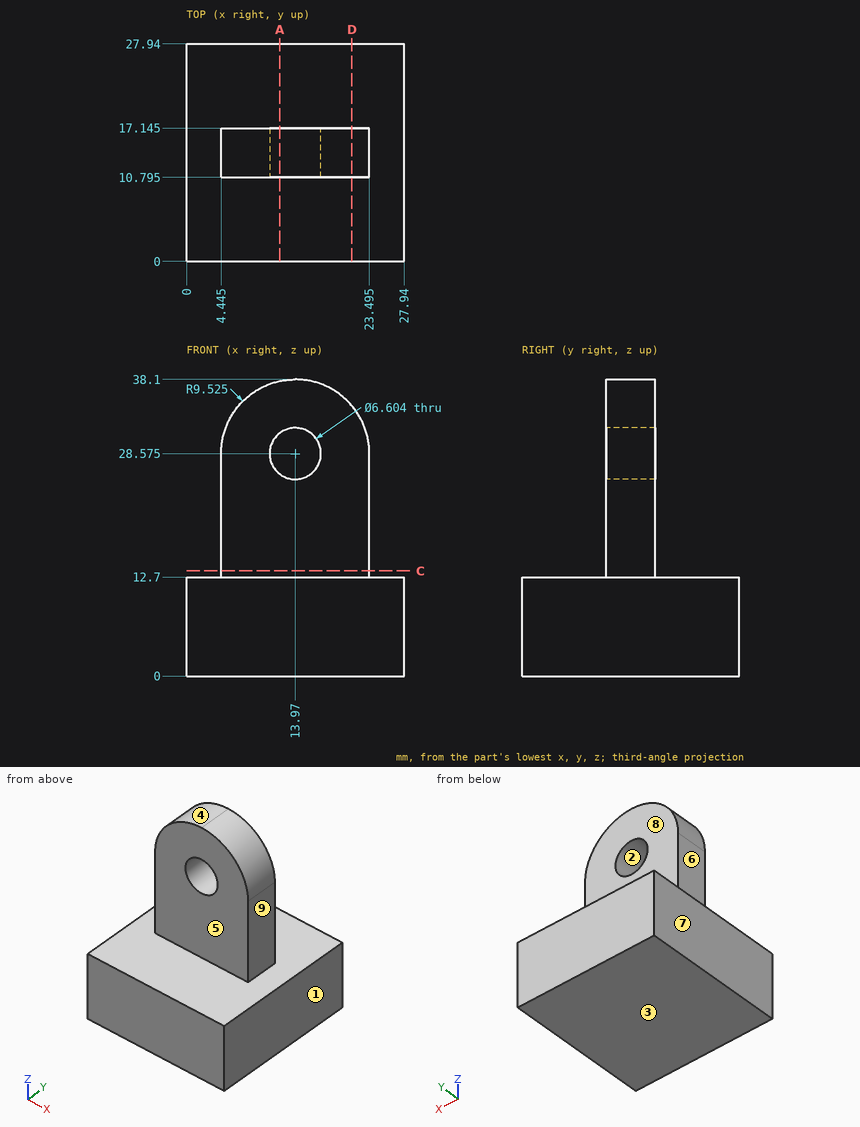
Study the drawing (mm; zero at the part's minimum x, y, z) and answer. A direction names the side the tool comes from. Give positions to 0.01 mm unless a question says otherwise; leave off trailing zeros. Loops run counter-clockwise (first coordinate to the right, second up) from the corner with the lowest first, then second, coordinate; pieces in that order, holes last. Notation, with made-up numbers: (82.25, 88) - (112.25, 88) arc R23 cw to (112.25, 113) - close; hole circle Ø2 at (-3, 52). An arc over 180 degrees is marked (long way). Return JSON: item names as keys, results as strings. Group by question number.
1. Straight lines are drawn through the part: line 1 (Z direction, x = 13.97, y = 14.75); line 2 (Y direction, x = 10.25, z = 31) (3 decimals); line 3 (Z direction, x = 9.75, y = 5.5). For each, find the intervals that lie inside material, in ascending order. Write a range as [from, to].
2. Which of the six approach directions +Z, -Z, +X, -X, +Y, -Y give full straight-line access (tool end or side, diameter ignored) to the marked faces 5, 6, 7, 8 and 9?
3. Given pin 1 Ø4 at (x, y) = (12.5, 7.5) entering from -Z; pin 2 Ø1.9 at (y, z) = (14, 21) entering from -X (3 decimals); pin 3 Ø4 at (x, y) = (19.5, 8) entering from +Z; pin 4 Ø5.5 at (x, z) = (15.5, 31) entering from -Y (3 decimals), each flat-ended and moving along its own axis, determine where each tip first touches the part or whether it passes through.
4. Find section D-D (x = 21.25). Write down the section's boundary in (y, z) (3 decimals).
5. Determine the mould class of the marked faces 1, 2, 3 and 4 for opening direction X: pulls with the +X half, pulls with the -X half, needs draft (parallel to the pull), parting line crosses it, or undercut.
6. Find section A-A (x = 12). Write down the section's boundary in (y, z) (3 decimals).
7. Find section C-C (z = 13.5). Write down the section's boundary in (x, y) (3 decimals).
Verdict:
{
 "1": {"line 1": "z = [0, 25.27], [31.88, 38.1]", "line 2": "y = [10.795, 17.145]", "line 3": "z = [0, 12.7]"},
 "2": {"face 5": "+Z, +X, -X, -Y", "face 6": "+Z, -X, +Y, -Y", "face 7": "+Z, -Z, -X, +Y, -Y", "face 8": "+Z, +X, -X, +Y", "face 9": "+Z, +X, +Y, -Y"},
 "3": {"pin 1": "stops at z = 0", "pin 2": "stops at x = 4.445", "pin 3": "stops at z = 12.7", "pin 4": "stops at y = 10.795"},
 "4": {"outline": "(0, 0) - (27.94, 0) - (27.94, 12.7) - (17.145, 12.7) - (17.145, 34.717) - (10.795, 34.717) - (10.795, 12.7) - (0, 12.7) - close"},
 "5": {"face 1": "pulls with the +X half", "face 2": "undercut", "face 3": "needs draft", "face 4": "pulls with the -X half"},
 "6": {"outline": "(0, 0) - (27.94, 0) - (27.94, 12.7) - (17.145, 12.7) - (17.145, 25.925) - (10.795, 25.925) - (10.795, 12.7) - (0, 12.7) - close; (10.795, 31.225) - (17.145, 31.225) - (17.145, 37.894) - (10.795, 37.894) - close"},
 "7": {"outline": "(4.445, 10.795) - (23.495, 10.795) - (23.495, 17.145) - (4.445, 17.145) - close"}
}
